from build123d import *

# Parameters (mm, degrees)
ESQUISSE1_W             = 30
ESQUISSE1_H             = 65
BOSS_EXTRU_1_DEPTH      = 6
ESQUISSE2_W             = 6
ESQUISSE2_H             = 10
BOSS_EXTRU_3_DEPTH      = 6
ESQUISSE3_R             = 2
ENL_V_MAT_EXTRU_1_DEPTH = 6


with BuildPart() as part:
    # Esquisse1 → Boss.-Extru.1 (new body)
    with BuildSketch(Plane.XY):
        with Locations((-15, 32.5)):
            Rectangle(ESQUISSE1_W, ESQUISSE1_H)
    extrude(amount=BOSS_EXTRU_1_DEPTH)

    # Esquisse2 → Boss.-Extru.3 (add)
    with BuildSketch(Plane(origin=(0, 0, 0), x_dir=(0, 0, -1), z_dir=(1, 0, 0))):
        with Locations((-3, 15)):
            Rectangle(ESQUISSE2_W, ESQUISSE2_H)
        with Locations((-3, 50)):
            Rectangle(ESQUISSE2_W, ESQUISSE2_H)
    extrude(amount=BOSS_EXTRU_3_DEPTH)

    # Esquisse3 → Enlèv. mat.-Extru.1 (cut)
    with BuildSketch(Plane.XY.offset(6)):
        with Locations((-25, 59)):
            Circle(ESQUISSE3_R)
        with Locations((-5, 59)):
            Circle(ESQUISSE3_R)
    extrude(amount=-ENL_V_MAT_EXTRU_1_DEPTH, mode=Mode.SUBTRACT)


solid = part.part
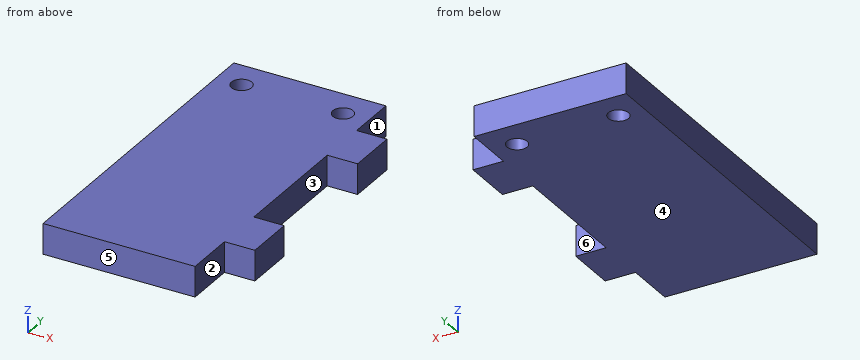
The listing builds one solid part. Answer for the finished solid, in the listing's coordinates (mm). Face numbers are marked on the shaded views. A direction names the side the tool comes from. Give positions to 0.01 mm unless a question says otherwise; leave off trailing zeros. Write each loop counter-clockwise with the first axis right and the second up, starting at its lowest first coordinate (ties: lowest second). Pieces come first, ordered by that corner, then holes. Notation, with made-up numbers: (69, -1.75) -> (84, -1.75) arc R20 ccw to (84, 21.25) -> close; hole circle Ø9 at (45, -6.75). An arc over 180 degrees is marked (long way). One line per question, with ' | ' between items. Start each with the question number.
1. Section D-D (x = -25) is taken. Determine the outline of the cut face in (y, z).
2. For the marked faces 1, 2 and 3, determine the directions among +Z, -Z, +X, -X, +Y, -Y from which every point of the face is accessible in a straight line to the end or side of a thin tool.
3. Section B-B (x = 1.5) is taken. Determine the outline of the cut face in (y, z), plus the area to 3 significant figures.
4. Find the intervals of material crossed by probe 1 along Y at (x, z) = (-25, 3.5); probe 2 along X at (y, z) = (58.5, 0.75); probe 3 along X at (y, z) = (41, 1.8), in increasing order.
5. For a pull along Y with two mould halves and no side action, classify the marked faces 4, 5 and 6 as pulls with the +Y half, pulls with the -Y half, needs draft (parallel to the pull), parting line crosses it, or undercut.
6. Section A-A (y = 59) is taken. Determine the outline of the cut face in (x, z).
7. Given pin 1 Ø1.8 at (x, z) = (1.5, 3.5) entering from -Y; pin 2 Ø1.8 at (y, z) = (62, 3.5) entering from +X; pin 3 Ø3 at (x, z) = (4, 4.5) entering from +Y, each flat-ended and moving along its own axis, determine where each tip first touches the part or whether it passes through.
8. Section C-C (z = 1.55) is taken. Determine the outline of the cut face in (x, y), plus the area to 3 significant figures.
Response values:
1) outline: (0, 0) -> (57, 0) -> (57, 6) -> (0, 6) -> close; (61, 0) -> (65, 0) -> (65, 6) -> (61, 6) -> close
2) face 1: +Z, -Z, +X, +Y | face 2: +Z, -Z, +X, -Y | face 3: +Z, -Z, +X
3) outline: (10, 0) -> (20, 0) -> (20, 6) -> (10, 6) -> close; (45, 0) -> (55, 0) -> (55, 6) -> (45, 6) -> close | area: 120 mm2
4) probe 1: 0 to 57, 61 to 65 | probe 2: -30 to -26.94, -23.06 to -6.94, -3.06 to 0 | probe 3: -30 to 0
5) face 4: needs draft | face 5: pulls with the -Y half | face 6: undercut
6) outline: (-30, 0) -> (-27, 0) -> (-27, 6) -> (-30, 6) -> close; (-23, 0) -> (-7, 0) -> (-7, 6) -> (-23, 6) -> close; (-3, 0) -> (0, 0) -> (0, 6) -> (-3, 6) -> close
7) pin 1: y = 10 | pin 2: x = 0 | pin 3: y = 55
8) outline: (-30, 0) -> (0, 0) -> (0, 10) -> (6, 10) -> (6, 20) -> (0, 20) -> (0, 45) -> (6, 45) -> (6, 55) -> (0, 55) -> (0, 65) -> (-30, 65) -> close; hole circle Ø4 at (-25, 59); hole circle Ø4 at (-5, 59) | area: 2,040 mm2
